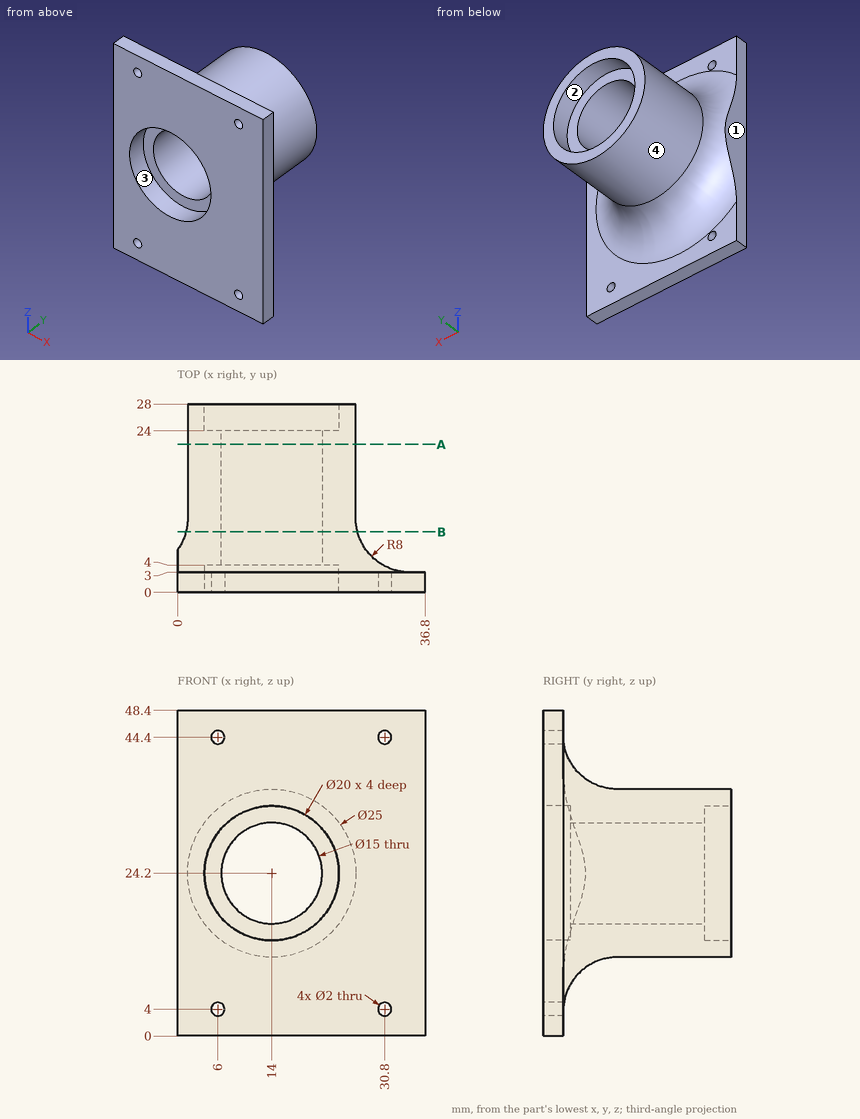
Could you check a few things on this drawing? It's one solid part, dimensions in mm from its lowest x, y, z. Coordinates: 2 decimals unless noted, no trailing zeros. Order: outer loops, then holes, each group sorted by start corner. A loop starts at its lowest first (then second) coordinate and runs counter-clockwise, first axis right, second up.
1. If we section it at A-A (y = 22): Please give me the cut outline in (x, z), then the cut area to 3 significant figures.
2. If we section it at B-B (y = 9): Please give me the cut outline in (x, z), then the cut area to 3 significant figures.
3. I'm going to push flat-ended pins straight in: pin 1 (6 mm diameter, centred on x = 11.5, z = 28, fed in from -Y); pin 2 (2.5 mm diameter, centred on x = 6, z = 4, fed in from +Y); pin 3 (6 mm diameter, centred on y = 19.5, z = 18.5, fed in from -X). Where does each tip first touch, or does it pass through?
4. I need wall thicknesses on line 1 (X direction, y = 0.7, z = 44.4); line 2 (Y direction, x = 12.5, z = 45); line 3 (Z direction, x = 11.5, y = 2). Which ranges of each line are inside material? Lowest first, please.
5. Thinking about a two-plate mould opening in Z: for the marked faces 1, 2, 3 and 4, which applies, +Z half, -Z half, draft (parallel to the pull), parting line (faces both ways), or undercut?
Entries:
1. outline: circle Ø25 at (14, 24.2); hole circle Ø15 at (14, 24.2)
1. area: 314 mm2
2. outline: circle Ø25.51 at (14, 24.2); hole circle Ø15 at (14, 24.2)
2. area: 334 mm2
3. pin 1: stops at y = 4
3. pin 2: stops at y = 3
3. pin 3: stops at x = 1.8
4. line 1: x = 0 to 5, 7 to 29.8, 31.8 to 36.8
4. line 2: y = 0 to 3
4. line 3: z = 0 to 14.52, 33.88 to 48.4
5. face 1: draft
5. face 2: undercut
5. face 3: undercut
5. face 4: parting line
